Autodesk Inventor part; units mm, degrees
ref_plane "YZ Plane" through (0, 0, 0) normal (1, 0, 0) x (0, 1, 0)
ref_plane "XZ Plane" through (0, 0, 0) normal (0, 1, 0) x (-1, 0, 0)
ref_plane "XY Plane" through (0, 0, 0) normal (0, 0, 1) x (1, 0, 0)
sketch "Sketch1" plane through (0, 0, 0) normal (0, 0, 1) x (1, 0, 0)
  line L0 (-46, -75) -> (46, -75)
  line L1 (46, -75) -> (46, 75)
  line L2 (46, 75) -> (-46, 75)
  line L3 (-46, 75) -> (-46, -75)
  line L4 (-46, -75) -> (46, 75) construction
  line L5 (46, -75) -> (-46, 75) construction
  point P0 (0, 0)
  dimension "d154" = 92
  dimension "d155" = 150
extrude "Plate5" add sketch "Sketch1" along normal blind 2
sketch "Sketch7" plane through (-44, -75, 0) normal (-1, 0, 0) x (0, -1, 0)
  line L0 (-150, 0) -> (0, 0)
  line L1 (0, 0) -> (0, 94)
  line L2 (0, 94) -> (-150, 94)
  line L3 (-150, 94) -> (-150, 0)
edge flange "Flange3" height 94 angle 90 thickness 2 bend radius 2.75 thickness toward (-1, 0, 0) relief round relief width 2 relief depth 1 edges at (-46, 0, 2) wall of the first edge with corners at (-44, 75, 0) (-44, -75, 0) (-44, -75, 94) (-44, 75, 94)
bend "Bend3"
corner "Corner3"
sketch "Sketch8" plane through (0, 0, 2) normal (0, 0, 1) x (1, 0, 0)
  line L0 (46, 75) -> (46, -75)
  line L1 (-41.25, 75) -> (46, 75)
  line L2 (32.375, 70) -> (-27.625, 70)
  line L3 (-27.625, 70) -> (-27.625, -26)
  line L4 (-27.625, -26) -> (32.375, -26)
  line L5 (32.375, -26) -> (32.375, 70)
  line L6 (32.375, 70) -> (-27.625, -26) construction
  line L7 (-27.625, 70) -> (32.375, -26) construction
  point P0 (0, 0)
  point P1 (2.375, 22)
  point P2 (2.375, 75)
  dimension "d167" = 60
  dimension "d168" = 96
  dimension "d169" = 5
extrude "Cut1" cut sketch "Sketch8" against normal blind 2
properties part number "PNS 1652 FDS Central tube wall" material "Stainless Steel"
The model under review builds one solid part; all positions refer to its coordinate system, in mm. A direction names the side the tool comes from. Round coordinates to 2 decimals unless told otherwise and drop trailing zeros. Write each loop counter-clockwise with the first axis right and the second up, starting at its lowest first coordinate (ties: lowest second). Pieces come first, ordered by that corner, then holes. Notation, with made-up numbers: (86, 88) - (129, 88) arc R24 cw to (129, 123) - close; hole circle Ø1 at (8, -26). An arc over 180 degrees is marked (long way). One line per item, written item: value. Start each with the question number.
1. Machinability: for faces 4 (the face through (-46, -1, 50)), 5 (the face through (2, -32, 2)), which of the approach directions +Z, -Z, +X, -X, +Y, -Y give a long, thin tool a straight path to every point of the face, cutting with its end or side? Answer none if there is none.
2. Clearance check with a flat-ended pin moving along its axis: P1, Ø0.6, axis at y = 1.5, z = 0.5, coming from the -X side. State where the tip first meets the part, or that it passes through.
3. Consider section A-A on y = 39. Write out the cut boundary in (x, z) (3 decimals).
4. To check wall thickness, follow L1, parallel to Z at x = -28, y = -51.5; L2, parallel to X at y = -37.5, z = 73. State the ranges of each line that lie inside material, in increasing order. Write a range as from..to.
5. Consider section C-C on y = -57.5. Write out the cut boundary in (x, z), and give its area (3 significant figures).
6. The part is to be moulded in two halves that separate along Y. For faces 1 (the face through (-45, 75, 26)), 2 (the face through (-44.645, -1.05, 1.428)), 3 (the face through (-45, -75, 26)), say which applies: released by +Y, released by -Y, zero draft, split by the parting line, or undercut.
7. Consider section D-D on x = 40.5. Write out the cut boundary in (y, z).
8. Consider section B-B on x = -2.5. Write out the cut boundary in (y, z), and give its area (3 significant figures).
Checks:
1. face 4: +Z, -Z, -X, +Y, -Y
1. face 5: +Z, +X, +Y, -Y
2. P1: stops at x = -43.89
3. outline: (-46, 4.75) arc R4.75 ccw to (-41.25, 0) - (-27.625, 0) - (-27.625, 2) - (-41.25, 2) arc R2.75 cw to (-44, 4.75) - (-44, 94) - (-46, 94) - close; (32.375, 0) - (46, 0) - (46, 2) - (32.375, 2) - close
4. L1: z = 0..2
4. L2: x = -46..-44
5. outline: (-46, 4.75) arc R4.75 ccw to (-41.25, 0) - (46, 0) - (46, 2) - (-41.25, 2) arc R2.75 cw to (-44, 4.75) - (-44, 94) - (-46, 94) - close
5. area: 365 mm^2
6. face 1: released by +Y
6. face 2: zero draft
6. face 3: released by -Y
7. outline: (-75, 0) - (75, 0) - (75, 2) - (-75, 2) - close
8. outline: (-75, 0) - (-26, 0) - (-26, 2) - (-75, 2) - close; (70, 0) - (75, 0) - (75, 2) - (70, 2) - close
8. area: 108 mm^2
